Could you check a few things on this model? Use its own coordinates, in mm. A direction names the side the tool comes from. Give positions to 0.01 mm unless a question says otherwise; leave off trailing zeros. Loops run counter-clockwise (first coordinate to the right, second up) from the corner with the lowest first, then second, coordinate; pieces in that order, holes last. Notation, with made-up numbers: M 16,11 L 23,11 A20 ccw 23,40 Z; hole C 71.5,67.5 d2. An arc over 180 degrees is marked long. Use CSV: the item, a comma, the result in double quotes.
```python
from build123d import *

# Parameters (mm, degrees)
SKETCH_1_W           = 15
SKETCH_1_H           = 15
SKETCH_1_W_2         = 12
SKETCH_1_H_2         = 12
EXTRUDE_2_DEPTH      = 174
SKETCH_3_R           = 1.5
CUT_EXTRUDE_2_DEPTH  = 10
SKETCH_6_R           = 4
CUT_EXTRUDE_4_DEPTH  = 10
SKETCH_7_R           = 1.5
CUT_EXTRUDE_5_DEPTH  = 10
SKETCH_8_R           = 4
CUT_EXTRUDE_6_DEPTH  = 10
SKETCH_10_R          = 1.5
CUT_EXTRUDE_9_DEPTH  = 10
SKETCH_13_R          = 1.5
CUT_EXTRUDE_11_DEPTH = 10
SKETCH_16_R          = 1.5
CUT_EXTRUDE_14_DEPTH = 10
SKETCH_17_R          = 6
CUT_EXTRUDE_15_DEPTH = 10
SKETCH_18_R          = 1.5
CUT_EXTRUDE_16_DEPTH = 10
SKETCH_19_R          = 4
CUT_EXTRUDE_17_DEPTH = 10
SKETCH_20_R          = 1.5
CUT_EXTRUDE_18_DEPTH = 10
SKETCH_21_R          = 1.5
CUT_EXTRUDE_19_DEPTH = 10
SKETCH_22_R          = 4
CUT_EXTRUDE_20_DEPTH = 10
SKETCH_23_R          = 1.5
CUT_EXTRUDE_21_DEPTH = 10
SKETCH_24_R          = 4
CUT_EXTRUDE_22_DEPTH = 10
SKETCH_25_R          = 4
CUT_EXTRUDE_23_DEPTH = 10
SKETCH_26_R          = 6
CUT_EXTRUDE_24_DEPTH = 10


with BuildPart() as part:
    # ｽｹｯﾁ1 → ﾎﾞｽ - 押し出し2 (new body)
    with BuildSketch(Plane.XY):
        with Locations((0.489915859, 0.232626086)):
            Rectangle(SKETCH_1_W, SKETCH_1_H)
        with Locations((0.489915859, 0.232626086)):
            Rectangle(SKETCH_1_W_2, SKETCH_1_H_2, mode=Mode.SUBTRACT)
    extrude(amount=EXTRUDE_2_DEPTH)

    # ｽｹｯﾁ3 → ｶｯﾄ - 押し出し2 (cut)
    with BuildSketch(Plane(origin=(7.989915859, 0, 0), x_dir=(0, 0, -1), z_dir=(1, 0, 0))):
        with Locations((-52.5, 0.232626086)):
            Circle(SKETCH_3_R)
    extrude(amount=-CUT_EXTRUDE_2_DEPTH, mode=Mode.SUBTRACT)

    # ｽｹｯﾁ6 → ｶｯﾄ - 押し出し4 (cut)
    with BuildSketch(Plane.ZY.offset(7.010084141)):
        with Locations((52.5, 0.232626086)):
            Circle(SKETCH_6_R)
    extrude(amount=-CUT_EXTRUDE_4_DEPTH, mode=Mode.SUBTRACT)

    # ｽｹｯﾁ7 → ｶｯﾄ - 押し出し5 (cut)
    with BuildSketch(Plane(origin=(7.989915859, 0, 0), x_dir=(0, 0, -1), z_dir=(1, 0, 0))):
        with Locations((-151.5, 0.232626086)):
            Circle(SKETCH_7_R)
    extrude(amount=-CUT_EXTRUDE_5_DEPTH, mode=Mode.SUBTRACT)

    # ｽｹｯﾁ8 → ｶｯﾄ - 押し出し6 (cut)
    with BuildSketch(Plane.ZY.offset(7.010084141)):
        with Locations((151.5, 0.232626086)):
            Circle(SKETCH_8_R)
    extrude(amount=-CUT_EXTRUDE_6_DEPTH, mode=Mode.SUBTRACT)

    # ｽｹｯﾁ10 → ｶｯﾄ - 押し出し9 (cut)
    with BuildSketch(Plane.ZY.offset(7.010084141)):
        with Locations((86.8, 0.232626086)):
            Circle(SKETCH_10_R)
    extrude(amount=-CUT_EXTRUDE_9_DEPTH, mode=Mode.SUBTRACT)

    # ｽｹｯﾁ13 → ｶｯﾄ - 押し出し11 (cut)
    with BuildSketch(Plane.ZY.offset(7.010084141)):
        with Locations((116.8, 0.232626086)):
            Circle(SKETCH_13_R)
    extrude(amount=-CUT_EXTRUDE_11_DEPTH, mode=Mode.SUBTRACT)

    # ｽｹｯﾁ16 → ｶｯﾄ - 押し出し14 (cut)
    with BuildSketch(Plane(origin=(0, 7.732626086, 0), x_dir=(1, 0, 0), z_dir=(0, 1, 0))):
        with Locations((0.489915859, -22.5)):
            Circle(SKETCH_16_R)
    extrude(amount=-CUT_EXTRUDE_14_DEPTH, mode=Mode.SUBTRACT)

    # ｽｹｯﾁ17 → ｶｯﾄ - 押し出し15 (cut)
    with BuildSketch(Plane.XZ.offset(7.267373914)):
        with Locations((0.489915859, 166.5)):
            Circle(SKETCH_17_R)
    extrude(amount=-CUT_EXTRUDE_15_DEPTH, mode=Mode.SUBTRACT)

    # ｽｹｯﾁ18 → ｶｯﾄ - 押し出し16 (cut)
    with BuildSketch(Plane(origin=(0, 7.732626086, 0), x_dir=(1, 0, 0), z_dir=(0, 1, 0))):
        with Locations((0.489915859, -166.5)):
            Circle(SKETCH_18_R)
    extrude(amount=-CUT_EXTRUDE_16_DEPTH, mode=Mode.SUBTRACT)

    # ｽｹｯﾁ19 → ｶｯﾄ - 押し出し17 (cut)
    with BuildSketch(Plane.ZY.offset(7.010084141)):
        with Locations((67.5, 0.232626086)):
            Circle(SKETCH_19_R)
    extrude(amount=-CUT_EXTRUDE_17_DEPTH, mode=Mode.SUBTRACT)

    # ｽｹｯﾁ20 → ｶｯﾄ - 押し出し18 (cut)
    with BuildSketch(Plane(origin=(7.989915859, 0, 0), x_dir=(0, 0, -1), z_dir=(1, 0, 0))):
        with Locations((-67.5, 0.232626086)):
            Circle(SKETCH_20_R)
    extrude(amount=-CUT_EXTRUDE_18_DEPTH, mode=Mode.SUBTRACT)

    # ｽｹｯﾁ21 → ｶｯﾄ - 押し出し19 (cut)
    with BuildSketch(Plane(origin=(7.989915859, 0, 0), x_dir=(0, 0, -1), z_dir=(1, 0, 0))):
        with Locations((-136.5, 0.232626086)):
            Circle(SKETCH_21_R)
    extrude(amount=-CUT_EXTRUDE_19_DEPTH, mode=Mode.SUBTRACT)

    # ｽｹｯﾁ22 → ｶｯﾄ - 押し出し20 (cut)
    with BuildSketch(Plane.ZY.offset(7.010084141)):
        with Locations((136.5, 0.232626086)):
            Circle(SKETCH_22_R)
    extrude(amount=-CUT_EXTRUDE_20_DEPTH, mode=Mode.SUBTRACT)

    # ｽｹｯﾁ23 → ｶｯﾄ - 押し出し21 (cut)
    with BuildSketch(Plane(origin=(0, 7.732626086, 0), x_dir=(1, 0, 0), z_dir=(0, 1, 0))):
        with Locations((0.489915859, -7.5)):
            Circle(SKETCH_23_R)
    extrude(amount=-CUT_EXTRUDE_21_DEPTH, mode=Mode.SUBTRACT)

    # ｽｹｯﾁ24 → ｶｯﾄ - 押し出し22 (cut)
    with BuildSketch(Plane(origin=(0, 7.732626086, 0), x_dir=(1, 0, 0), z_dir=(0, 1, 0))):
        with Locations((0.489915859, -86.8)):
            Circle(SKETCH_24_R)
    extrude(amount=-CUT_EXTRUDE_22_DEPTH, mode=Mode.SUBTRACT)

    # ｽｹｯﾁ25 → ｶｯﾄ - 押し出し23 (cut)
    with BuildSketch(Plane(origin=(0, 7.732626086, 0), x_dir=(1, 0, 0), z_dir=(0, 1, 0))):
        with Locations((0.489915859, -116.8)):
            Circle(SKETCH_25_R)
    extrude(amount=-CUT_EXTRUDE_23_DEPTH, mode=Mode.SUBTRACT)

    # ｽｹｯﾁ26 → ｶｯﾄ - 押し出し24 (cut)
    with BuildSketch(Plane.XZ.offset(7.267373914)):
        with Locations((0.489915859, 22.5)):
            Circle(SKETCH_26_R)
    extrude(amount=-CUT_EXTRUDE_24_DEPTH, mode=Mode.SUBTRACT)


solid = part.part
```
1. Which directions (+Z, -Z, +X, -X, +Y, -Y) give clear straight access to the entire face, cutting with the end or side of a thin tool? Please do faces 5 (the face through (-0.811, -6.528, 16.643)), 6 (the face through (-6.271, 2.936, 133.552)), 7 (the face through (0, -5.767, 9)), 8 (the face through (2.336, 6.993, 90.349)).
Outcome:
face 5,"-Y"
face 6,"-X"
face 7,"+Z, -Z"
face 8,"+Y"
2. I want a section at A-A, the plane z = 86.8. List the corners of the cut face in (x, y) for me.
Outcome:
outline,"M -7.01,-7.27 L 7.99,-7.27 L 7.99,7.73 L 4.49,7.73 L 4.49,6.23 L 6.49,6.23 L 6.49,-5.77 L -5.51,-5.77 L -5.51,-1.27 L -7.01,-1.27 Z; M -7.01,1.73 L -5.51,1.73 L -5.51,6.23 L -3.51,6.23 L -3.51,7.73 L -7.01,7.73 Z"
3. I'm going to push flat-ended pins straight in: pin 1 Ø4 at (x, y) = (2.5, 2) entering from -Z; pin 2 Ø5 at (x, z) = (0.49, 86.8) entering from +Y; pin 3 Ø3.5 at (y, z) = (0.23, 52.5) entering from -X. Where does each tip first touch, or does it pass through?
Outcome:
pin 1,"through"
pin 2,"y = -5.77"
pin 3,"x = 6.49"
4. Please list where these lines run through material, in increasing order: line 1 (X direction, y = -1.5, z = 110); line 2 (Y direction, x = 4, z = 49); line 3 (Y direction, x = -6.2, z = 86.8).
Outcome:
line 1,"-7.01 to -5.51, 6.49 to 7.99"
line 2,"-7.27 to -5.77, 6.23 to 7.73"
line 3,"-7.27 to -1.27, 1.73 to 7.73"
5. If we mould it in two halves opening along X, with no side actions, what happens to faces 1 (the face through (-4, 6.233, 86)), 2 (the face through (-0.4, 7, 120.7)), 3 (the face through (7.99, 0, 86)), 4 (the face through (-6, 0, 174))? For each: +X half, -X half, draft (parallel to the pull), parting line (faces both ways), or undercut.
Outcome:
face 1,"undercut"
face 2,"undercut"
face 3,"+X half"
face 4,"draft"
